Can you work these out from the model? Positions are in its coordinate system, mm. A direction names the side the tool comes from. Round coordinates to 2 decimals unless told otherwise and drop trailing zeros. Loops run counter-clockwise (first coordinate to the right, second up) from the corner with the lowest first, then second, coordinate; pieces in that order, holes last.
from build123d import *

# Parameters (mm, degrees)
BOSS_EXTRUDE2_DEPTH = 25
CUT_EXTRUDE2_DEPTH  = 35
FILLET3_R           = 10
SKETCH5_R           = 14.294796693
CUT_EXTRUDE3_DEPTH  = 15
FILLET4_R           = 10
FILLET5_R           = 5
SKETCH6_R           = 6
CUT_EXTRUDE4_DEPTH  = 35
SKETCH8_W           = 35
SKETCH8_H           = 26.166184444
CUT_EXTRUDE6_DEPTH  = 10.066320609
SCALE1_SCALE        = 0.25


with BuildPart() as part:
    # Sketch2 → Boss-Extrude2 (new, symmetric)
    with BuildSketch(Plane(origin=(0, 0, 0), x_dir=(0, 0, -1), z_dir=(1, 0, 0))):
        Polygon((-62.071067812, 55), (-62.071067812, -5), (-92.071067812, -5), (-92.071067812, -17.136235823), (92.071067812, -17.136235823), (92.071067812, -5), (62.071067812, -5), (62.071067812, 55), align=None)
    extrude(amount=BOSS_EXTRUDE2_DEPTH, both=True)

    # Sketch3 → Cut-Extrude2 (cut)
    with BuildSketch(Plane(origin=(25, 0, 0), x_dir=(0, 0, -1), z_dir=(1, 0, 0))):
        Polygon((0, -15.066320609), (60, 44.933679391), (-60, 44.933679391), align=None)
    extrude(amount=-CUT_EXTRUDE2_DEPTH, mode=Mode.SUBTRACT)

    # Fillet3
    fillet3_edges = [part.edges().sort_by_distance(p)[0] for p in [
        (7.5, -15.066320609, 0),
        (7.5, 44.933679391, 60),
        (7.5, 44.933679391, -60),
    ]]
    fillet(fillet3_edges, radius=FILLET3_R)

    # Sketch5 → Cut-Extrude3 (cut)
    with BuildSketch(Plane(origin=(-10, 0, 0), x_dir=(0, 0, -1), z_dir=(1, 0, 0))):
        with Locations((0, -0.924184985)):
            Circle(SKETCH5_R)
    extrude(amount=-CUT_EXTRUDE3_DEPTH, mode=Mode.SUBTRACT)

    # Fillet4
    fillet4_edges = [part.edges().sort_by_distance(p)[0] for p in [
        (0, 55, 62.071067812),
        (0, 55, -62.071067812),
    ]]
    fillet(fillet4_edges, radius=FILLET4_R)

    # Fillet5
    fillet5_edges = [part.edges().sort_by_distance(p)[0] for p in [
        (0, -5, -62.071067812),
        (0, -5, 62.071067812),
    ]]
    fillet(fillet5_edges, radius=FILLET5_R)

    # Sketch6 → Cut-Extrude4 (cut)
    with BuildSketch(Plane(origin=(0, -5, 0), x_dir=(1, 0, 0), z_dir=(0, 1, 0))):
        with Locations(Location((-12.273124469, -79.571067812, 0), (0, 0, 270))):
            Circle(SKETCH6_R)
        with Locations(Location((12.273124469, -79.571067812, 0), (0, 0, 270))):
            Circle(SKETCH6_R)
    cut_extrude4 = extrude(amount=-CUT_EXTRUDE4_DEPTH, mode=Mode.SUBTRACT)

    # Mirror1: Cut-Extrude4 across plane
    add(cut_extrude4.mirror(Plane.XY), mode=Mode.SUBTRACT)

    # Sketch8 → Cut-Extrude6 (cut)
    with BuildSketch(Plane(origin=(0, 55, 0), x_dir=(1, 0, 0), z_dir=(0, 1, 0))):
        with Locations((7.5, 0)):
            Rectangle(SKETCH8_W, SKETCH8_H)
    extrude(amount=-CUT_EXTRUDE6_DEPTH, mode=Mode.SUBTRACT)


with BuildPart() as part_1:
    # Scale1: scaled about (-2.268878972, 13.955162183, 0)
    add(part.part.scale(SCALE1_SCALE).moved(Location((-1.701659229, 10.466371637, 0))))


solid = part_1.part
(1) If we mould it in two halves opening along Y, with no side actions, what happens to faces 1 (the cylindrical face through (-6.05, 6.747, 0.775)), 2 (the flat face through (4.548, 11, -5)), 3 (the flat face through (-2, 6.182, 0)), 4 (the flat face through (-4.4, 24.216, -0.2))? For each: released by +Y, released by -Y, zero draft, split by the parting line, or undercut.
Worked answers:
face 1: undercut
face 2: zero draft
face 3: released by -Y
face 4: released by +Y
(2) For faces 5 (the flat face through (0, 23, 3.271)), 6 (the flat face through (0, 21.7, 6)), 7 (the flat face through (-2, 9.216, -20)), 8 (the flat face through (-4.202, 7.5, -0.2)), which set-ups out of +Z, -Z, +X, -X, +Y, -Y let a thin tool reach every point of the face, with its end or its side?
Worked answers:
face 5: +X, +Y
face 6: +X
face 7: -Z, +X, -X, +Y
face 8: -X
(3) If I drill on line 1 (Y direction, x = -6, z = 0); line 2 (Z direction, x = 2.5, y = 8); line 3 (Z direction, x = -7, y = 19.5), over which ranges is the centre line in solid material (lowest first)?
Worked answers:
line 1: y = 6.18 to 6.66, 13.81 to 24.22
line 2: z = -23.02 to -20.88, -18.91 to -1.12, 1.12 to 18.91, 20.88 to 23.02
line 3: z = -15.52 to 15.52
(4) If we section it at D-D, the plane y = 19: List the corners of the cut face in (x, z) for me.
Worked answers:
outline: (-7.95, -15.52) - (4.55, -15.52) - (4.55, -11.46) - (-4.2, -11.46) - (-4.2, 11.46) - (4.55, 11.46) - (4.55, 15.52) - (-7.95, 15.52) - close
(5) If we section it at B-B, the plane x = -5.5: List the corners of the cut face in (y, z) for me, then the cut area to 3 significant figures.
Worked answers:
outline: (6.18, -23.02) - (9.22, -23.02) - (9.22, -21.2) - (6.18, -21.2) - close; (6.18, -18.58) - (9.22, -18.58) - (9.22, -16.77) arc R1.25 cw to (10.47, -15.52) - (21.72, -15.52) arc R2.5 ccw to (24.22, -13.02) - (24.22, 13.02) arc R2.5 ccw to (21.72, 15.52) - (10.47, 15.52) arc R1.25 cw to (9.22, 16.77) - (9.22, 18.58) - (6.18, 18.58) - close; (6.18, 21.2) - (9.22, 21.2) - (9.22, 23.02) - (6.18, 23.02) - close; hole circle Ø7.15 at (10.24, 0)
area: 547 mm2
(6) If we section it at C-C, the plane x = -1: List the corners of the cut face in (y, z) for me, then the cut area to 3 significant figures.
Worked answers:
outline: (6.18, -23.02) - (9.22, -23.02) - (9.22, -16.77) arc R1.25 cw to (10.47, -15.52) - (21.72, -15.52) arc R2.5 ccw to (24.22, -13.02) - (24.22, -3.27) - (21.7, -3.27) - (21.7, -8.96) arc R2.5 cw to (17.43, -10.73) - (8.47, -1.77) arc R2.5 cw to (8.47, 1.77) - (17.43, 10.73) arc R2.5 cw to (21.7, 8.96) - (21.7, 3.27) - (24.22, 3.27) - (24.22, 13.02) arc R2.5 ccw to (21.72, 15.52) - (10.47, 15.52) arc R1.25 cw to (9.22, 16.77) - (9.22, 23.02) - (6.18, 23.02) - close
area: 379 mm2
(7) If we section it at A-A, the plane z = 0: List the corners of the cut face in (x, y) for me, then the cut area to 3 significant figures.
Worked answers:
outline: (-7.95, 6.18) - (4.55, 6.18) - (4.55, 7.74) - (-4.2, 7.74) - (-4.2, 6.66) - (-7.95, 6.66) - close; (-7.95, 13.81) - (-4.2, 13.81) - (-4.2, 24.22) - (-7.95, 24.22) - close
area: 54.4 mm2
(8) Will these pins go through, and if not, where does the flat tip stop? P1, Ø1, axis at x = -5, y = 12, coming from the -Z side; P2, Ø0.8, axis at x = -0.5, y = 23, coming from the -Z side; P3, Ø1.3, axis at x = -0.5, y = 23, coming from the +Z side.
Worked answers:
P1: stops at z = -15.52
P2: stops at z = -15.36
P3: stops at z = 15.44
